Autodesk Inventor part; units mm, degrees
ref_plane "Work Plane1" through (0, 0, 14) normal (0, 0, 1) x (1, 0, 0)
ref_plane "YZ Plane" through (0, 0, 0) normal (1, 0, 0) x (0, 1, 0)
ref_plane "XZ Plane" through (0, 0, 0) normal (0, 1, 0) x (-1, 0, 0)
sketch "Sketch1" plane through (0, 0, 0) normal (0, 0, 1) x (1, 0, 0)
  circle A0 centre (0, 0) radius 11
  dimension "d0" = 22
extrude "Extrusion1" add sketch "Sketch1" along normal blind 19
ref_plane "Work Plane1" through (0, 0, 14) normal (0, 0, 1) x (1, 0, 0)
sketch "Sketch2" plane through (0, 0, 14) normal (0, 0, 1) x (1, 0, 0)
  circle A0 centre (0, 0) radius 22.25
  circle A1 centre (0, 17.5) radius 2.5
  circle A2 centre (-15.1554, -8.75) radius 2.5
  circle A3 centre (15.1554, -8.75) radius 2.5
  dimension "d4" = 44.5
  dimension "d5" = 5
  dimension "d6" = 17.5
  dimension "d9" = 360
extrude "Extrusion2" add sketch "Sketch2" against normal blind 2.3
sketch "Sketch3" plane through (0, 0, 19) normal (0, 0, 1) x (1, 0, 0)
  circle A0 centre (0, 0) radius 3.5
  dimension "d13" = 7
extrude "Extrusion3" add sketch "Sketch3" along normal blind 7
properties part number "Slip Ring" material "ABS Plastic"
Can you work these out from the model? Positions are in its coordinate system, mm. A direction names the side the tool comes from. Give positions to 0.01 mm unless a question says otherwise; leave off trailing zeros. Order: outer loops, then holes, each group sorted by start corner. A loop starts at its lowest first (then second) coordinate and runs counter-clockwise, first axis right, second up. Notation, with made-up numbers: M -28.75,51.5 L 4.25,51.5 A20 cw 4.25,81.5 Z; hole C 32,56.5 d1. An arc over 180 degrees is marked long. One line per item, written item: value.
1) On a 3-axis mill with a long thin cutter (end or side, diameter ignored), from which of +Z, -Z, +X, -X, +Y, -Y can I reach the whole of each face in a straight line? I mean faces 4 (the face through (0, 0, 26)), 5 (the face through (3.233, 1.341, 22.451)), 6 (the face through (5, 10, 11.7)). Say none if no direction works.
Answer sheet:
face 4: +Z, +X, -X, +Y, -Y
face 5: +Z
face 6: -Z
2) I want a section at B-B, the plane y = -8.75. List the corners of the cut face in (x, z) for me.
Answer sheet:
outline: M -20.46,11.7 L -17.66,11.7 L -17.66,14 L -20.46,14 Z; M -12.66,11.7 L -6.67,11.7 L -6.67,0 L 6.67,0 L 6.67,11.7 L 12.66,11.7 L 12.66,14 L 6.67,14 L 6.67,19 L -6.67,19 L -6.67,14 L -12.66,14 Z; M 17.66,11.7 L 20.46,11.7 L 20.46,14 L 17.66,14 Z
3) Please list where these lines run through material, in increasing order: line 1 along Y through (x, z) = (0, 12.3); line 2 along Z through (x, y) = (13, 11); line 3 along Z through (x, y) = (9.5, -2).
Answer sheet:
line 1: y = -22.25 to 15, 20 to 22.25
line 2: z = 11.7 to 14
line 3: z = 0 to 19
4) For P1, Ø12, axis at x = 6, y = 4, coming from the +Z side; P2, Ø6.5, axis at x = 0, y = 17.5, coming from the -Z side; P3, Ø8, axis at y = -11.5, z = 4.5, coming from the +X side; P4, Ø4, axis at x = 6, z = 12.5, coming from the -Y side, each with a flat end and sliding along its axis, tell me the tip position at first contact or that it passes through.
Answer sheet:
P1: stops at z = 26
P2: stops at z = 11.7
P3: stops at x = 8.05
P4: stops at y = -21.89
5) We'd pull the mould along X, two halves only. Please class faces 1 (the face through (-3, 3, 19)), 2 (the face through (16.309, -10.968, 12.866)), 3 (the face through (-2.38, 10.74, 16.46)): released by +X, released by -X, zero draft, split by the parting line, or undercut.
Answer sheet:
face 1: zero draft
face 2: undercut
face 3: split by the parting line
6) I want a section at C-C, the plane y = 0. List the corners of the cut face in (x, z) for me.
Answer sheet:
outline: M -22.25,11.7 L -11,11.7 L -11,0 L 11,0 L 11,11.7 L 22.25,11.7 L 22.25,14 L 11,14 L 11,19 L 3.5,19 L 3.5,26 L -3.5,26 L -3.5,19 L -11,19 L -11,14 L -22.25,14 Z
7) I want a section at D-D, the plane z = 9. List the corners of the cut face in (x, y) for me, plus the area to 3 significant figures.
Answer sheet:
outline: C 0,0 d22
area: 380 mm^2
8) I want a section at A-A, the plane x = 0. List the corners of the cut face in (y, z) for me.
Answer sheet:
outline: M -22.25,11.7 L -11,11.7 L -11,0 L 11,0 L 11,11.7 L 15,11.7 L 15,14 L 11,14 L 11,19 L 3.5,19 L 3.5,26 L -3.5,26 L -3.5,19 L -11,19 L -11,14 L -22.25,14 Z; M 20,11.7 L 22.25,11.7 L 22.25,14 L 20,14 Z
